```python
from build123d import *

# Parameters (mm, degrees)
F0_W     = 60
F0_H     = 25
F1_DEPTH = 18
F3_DEPTH = 30
F4_R     = 3


# Not quite as in the source:
# - a feature names something its author has since deleted; it is built from what else it names


with BuildPart() as f1:
    # F0 (on Front) → F1 (new body)
    with BuildSketch(Plane.XZ):
        Rectangle(F0_W, F0_H)
    extrude(amount=F1_DEPTH)

    # F2 (on Right) → F3 (cut, symmetric)
    with BuildSketch(Plane.YZ):
        Polygon((0, 12.5), (-14.4337567297, 12.5), (-11.5470053838, 7.5), (0, -12.5), (0, 0), align=None)
        Polygon((-14.4337567297, 7.5), (-14.4337567297, 12.5), (-17.3205080757, 12.5), (-19.7896268219, 12.5), (-19.7896268219, -12.5), (-17.3205080757, -12.5), (-14.4337567297, -12.5), align=None)
        Polygon((-11.5470053838, 7.5), (-14.4337567297, 12.5), (-14.4337567297, 7.5), align=None)
    extrude(amount=F3_DEPTH, both=True, mode=Mode.SUBTRACT)

    # F4
    f4_edges = [f1.edges().sort_by_distance(p)[0] for p in [
        (30, -7.216878, -12.5),
        (-30, -7.216878, -12.5),
        (0, -14.433757, -12.5),
        (30, -14.433757, -2.5),
        (-30, -14.433757, -2.5),
    ]]
    fillet(f4_edges, radius=F4_R)


solid = f1.part
```
Part model, mm, in its own coordinate system. Coordinates: 2 decimals unless noted, no trailing zeros. Loops run counter-clockwise (first coordinate to the right, second up) from the corner with the lowest first, then second, coordinate; pieces in that order, holes last. Notation, with made-up numbers: (42.5, -36) - (88.5, -36) arc R13 cw to (88.5, -17) - close; hole circle Ø3 at (83, 3.5). An arc over 180 degrees is marked (long way). Write item = value, one per line. Start each with the question number.
Item 1: Cut at C-C, the plane y = -6.5. Give the cut face in (x, z).
Item 2: Flat gauge pins, fed straight in: pin 1 Ø4 at (x, z) = (6.5, -0.5) entering from +Y; pin 2 Ø8 at (x, y) = (-5, -2.5) entering from +Z. Where does each tip first touch, or does it go through?
Item 3: Cut at B-B, the plane z = -4. Give the cut face in (x, y).
Item 4: Wall check: L1, parallel to Y at x = -1.5, z = 2.5; L2, parallel to Y at x = -5, z = -9.5; L3, parallel to Z at x = -25, y = -5.5. Give the ranges that are in metal, low to high. Write a range as from..to.
Item 5: Cut at D-D, the plane y = -0.75. Give the cut face in (x, z), and give its area (3 significant figures).
Item 6: Cut at A-A, the plane x = -17.5. Give the cut face in (y, z), and give its area (3 significant figures).
The answers:
q1.outline = (-30, -9.5) arc R3 ccw to (-27, -12.5) - (27, -12.5) arc R3 ccw to (30, -9.5) - (30, -1.24) - (-30, -1.24) - close
q2.pin_1 = -5.77
q2.pin_2 = -1.24
q3.outline = (-30, -11.43) arc R3 ccw to (-27, -14.43) - (27, -14.43) arc R3 ccw to (30, -11.43) - (30, -4.91) - (-30, -4.91) - close
q4.L1 = -14.43..-8.66
q4.L2 = -14.43..-1.73
q4.L3 = -12.5..-2.97
q5.outline = (-29.47, -11.2) arc R3 ccw to (-27, -12.5) - (27, -12.5) arc R3 ccw to (29.47, -11.2) - close
q5.area = 74.7 mm2
q6.outline = (-14.43, -9.5) arc R3 ccw to (-11.43, -12.5) - (0, -12.5) - (-11.55, 7.5) - (-14.43, 7.5) - close
q6.area = 171 mm2
